Input: part model. Units: mm. Frame: model coordinates. A direction names the side the tool comes from. Coordinates: 2 decimals unless noted, no trailing zeros. Order: outer loops, then holes, each group sorted by start corner. A loop starts at its lowest first (then second) coordinate and runs counter-clockwise, first axis right, second up. Notation, with made-up numbers: (60.25, 72) - (74.25, 72) arc R30 ccw to (74.25, 95) - close; hole circle Ø1 at (83, -38). An arc over 180 degrees is marked (long way). One line per question, with ' | ' between items. Start each with the question number.
```python
from build123d import *

# Parameters (mm, degrees)
AUFSATZ_LINEAR_AUSTRAGEN1_DEPTH = 10
SCHNITT_LINEAR_AUSTRAGEN1_REACH = 218.035
SKIZZE2_W                       = 12.4
SKIZZE2_H                       = 5
VERRUNDUNG1_R                   = 0.5


with BuildPart() as part:
    # Skizze1 → Aufsatz-Linear austragen1 (new body)
    with BuildSketch(Plane.XY):
        with BuildLine():
            Line((-59.5275, -41.5905), (-73.15, -41.5905))
            Line((-73.15, -41.5905), (-85.55, -41.5905))
            Line((-85.55, -41.5905), (-169.0581, -41.5905))
            ThreePointArc((-169.0581, -41.5905), (-176.514207067, -44.783915623), (-179.34742314, -52.3842))
            Line((-179.34742314, -52.3842), (-179.34742314, -150.803560266))
            ThreePointArc((-179.34742314, -150.803560266), (-176.514004305, -158.403485592), (-169.0581, -161.5967))
            Line((-169.0581, -161.5967), (-59.5275, -161.5967))
            ThreePointArc((-59.5275, -161.5967), (-52.244300154, -158.579899846), (-49.2275, -151.2967))
            Line((-49.2275, -151.2967), (-49.2275, -51.8905))
            ThreePointArc((-49.2275, -51.8905), (-52.244300154, -44.607300154), (-59.5275, -41.5905))
        make_face()
        Polygon((-174.462899882, -152.4967), (-171.231946398, -152.4967), (-169.94742314, -155.0967), (-171.231946398, -157.6967), (-174.462899882, -157.6967), (-175.74742314, -155.0967), align=None, mode=Mode.SUBTRACT)
        Polygon((-58.1338, -155.0967), (-56.849276742, -152.4967), (-53.618323258, -152.4967), (-52.3338, -155.0967), (-53.618323258, -157.6967), (-56.849276742, -157.6967), align=None, mode=Mode.SUBTRACT)
        Polygon((-175.74742314, -48.0905), (-174.462899882, -45.4905), (-171.231946398, -45.4905), (-169.94742314, -48.0905), (-171.231946398, -50.6905), (-174.462899882, -50.6905), align=None, mode=Mode.SUBTRACT)
        with BuildLine():
            Line((-85.55, -51.0905), (-73.15, -51.0905))
            Line((-73.15, -51.0905), (-59.5275, -51.0905))
            ThreePointArc((-59.5275, -51.0905), (-58.612715957, -51.469415957), (-58.2338, -52.3842))
            Line((-58.2338, -52.3842), (-58.2338, -150.803))
            ThreePointArc((-58.2338, -150.803), (-58.612715957, -151.717784043), (-59.5275, -152.0967))
            Line((-59.5275, -152.0967), (-169.0581, -152.0967))
            ThreePointArc((-169.0581, -152.0967), (-169.972884043, -151.717784043), (-170.3518, -150.803))
            Line((-170.3518, -150.803), (-170.3518, -52.3842))
            ThreePointArc((-170.3518, -52.3842), (-169.972884043, -51.469415957), (-169.0581, -51.0905))
            Line((-169.0581, -51.0905), (-85.55, -51.0905))
        make_face(mode=Mode.SUBTRACT)
        Polygon((-58.1338, -48.0905), (-56.849276742, -45.4905), (-53.618323258, -45.4905), (-52.3338, -48.0905), (-53.618323258, -50.6905), (-56.849276742, -50.6905), align=None, mode=Mode.SUBTRACT)
    extrude(amount=AUFSATZ_LINEAR_AUSTRAGEN1_DEPTH)

    # Skizze2 → Schnitt-Linear austragen1 (cut, up to next)
    with BuildSketch(Plane(origin=(0, -41.5905, 0), x_dir=(1, 0, 0), z_dir=(0, 1, 0)), mode=Mode.PRIVATE) as schnitt_linear_austragen1_sk1:
        with Locations((-79.35, -2.5)):
            Rectangle(SKIZZE2_W, SKIZZE2_H)
    schnitt_linear_austragen1_tool1 = extrude(schnitt_linear_austragen1_sk1.sketch, amount=-SCHNITT_LINEAR_AUSTRAGEN1_REACH, mode=Mode.PRIVATE) & part.part
    add(schnitt_linear_austragen1_tool1.solids().sort_by_distance((-79.35, -41.5905, 2.5))[0], mode=Mode.SUBTRACT)

    # Verrundung1
    verrundung1_edges = [part.edges().sort_by_distance(p)[0] for p in [
        (-85.55, -46.3405, 5),
        (-73.15, -46.3405, 5),
    ]]
    fillet(verrundung1_edges, radius=VERRUNDUNG1_R)


solid = part.part
```
(1) Draft query along Y for faces 1 (the face through (-173, -157.697, 5)), 2 (the face through (-52.16, -44.69, 4.93)), 3 (the face through (-79, -46, 5)). Return one class per face: +Y half, -Y half, draft (parallel to the pull), parting line (faces both ways), or undercut.
(2) Section B-B (y = -139). Output: boundary loops of the cut face in (x, z).
(3) Pin query (flat end, axial travel): pin 1 (2.5 mm diameter, centred on x = -173.5, z = 6.5, fed in from +Y); pin 2 (3.5 mm diameter, centred on x = -173, z = 6.5, fed in from +Y); pin 3 (3 mm diameter, centred on y = -81.5, z = 5, fed in from -X). Return the tip coordinate at first contact, or that it passes through.
(4) Section A-A (x = -77.5). Output: boundary loops of the cut face in (y, z), then the cut area to 4 significant figures.
(5) Reachability of faces 4 (the face through (-55, -50.69, 5)), 5 (the face through (-115, -161.597, 5)) from +Z, -Z, +X, -X, +Y, -Y: full face, straight path, thin tool, end or side. Return the list, or none.
(6) Section C-C (z = 8). State how many separate pieces and enclosed holes the cut face has, then the cut area to 3 significant figures.
(7) Material intervals for line 1 along X through (y, z) = (-124.5, 4.5); line 2 along Y through (x, z) = (-87.5, 5); line 3 along Y through (x, z) = (-171.5, 1.25), sorted ascending. Write a range as from..to.
Worked answers:
1) face 1: undercut | face 2: +Y half | face 3: draft
2) outline: (-179.35, 0) - (-170.35, 0) - (-170.35, 10) - (-179.35, 10) - close; (-58.23, 0) - (-49.23, 0) - (-49.23, 10) - (-58.23, 10) - close
3) pin 1: stops at y = -42.1 | pin 2: stops at y = -41.83 | pin 3: stops at x = -179.35
4) outline: (-161.6, 0) - (-152.1, 0) - (-152.1, 10) - (-161.6, 10) - close; (-51.09, 5) - (-41.59, 5) - (-41.59, 10) - (-51.09, 10) - close | area: 142.5 mm²
5) face 4: +Z, -Z | face 5: +Z, -Z, +X, -X, -Y
6) separate pieces: 1 | enclosed holes: 5 | area: 4,110 mm²
7) line 1: x = -179.35..-170.35, -58.23..-49.23 | line 2: y = -161.6..-152.1, -51.09..-41.59 | line 3: y = -161.3..-157.7, -152.5..-50.69, -45.49..-41.88
